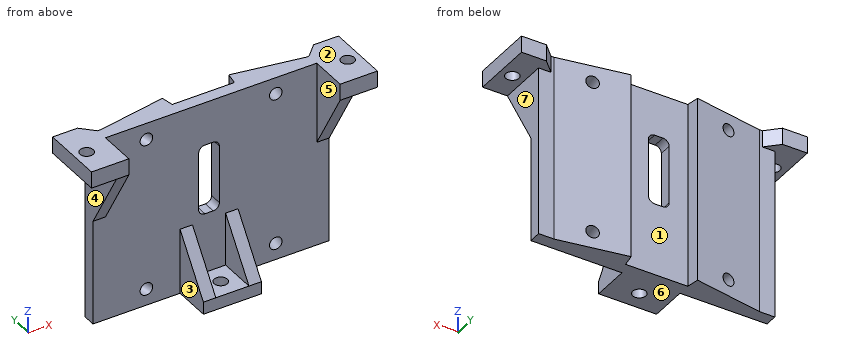
from build123d import *

# Parameters (mm, degrees)
SKETCH_1_W          = 57
SKETCH_1_H          = 45
EXTRUDE_1_DEPTH     = 3
SKETCH_2_W          = 4
SKETCH_2_H          = 15
EXTRUDE_2_DEPTH     = 6
SKETCH_3_W          = 4
SKETCH_3_H          = 15
EXTRUDE_3_DEPTH     = 6
EXTRUDE_4_DEPTH     = 3
SKETCH_5_W          = 4
SKETCH_5_H          = 9
EXTRUDE_5_DEPTH     = 3
CHAMFER_1_SIZE      = 3
SKETCH_6_R          = 1.6
CUT_EXTRUDE_1_DEPTH = 4
SKETCH_8_W          = 8
SKETCH_8_H          = 3
EXTRUDE_6_DEPTH     = 9
EXTRUDE_7_DEPTH     = 3
EXTRUDE_8_DEPTH     = 3
SKETCH_11_R         = 1.6
CUT_EXTRUDE_3_DEPTH = 3
SKETCH_12_W         = 5
SKETCH_12_H         = 17
CUT_EXTRUDE_4_DEPTH = 3
FILLET_1_R          = 1.5
EXTRUDE_9_REACH     = 80.57
SKETCH_15_W         = 45
SKETCH_15_H         = 17.726539555
SKETCH_16_R         = 1.5
CUT_EXTRUDE_5_DEPTH = 79.570276896


with BuildPart() as part:
    # 草图1 → 凸台-拉伸1 (new body)
    with BuildSketch(Plane(origin=(0, 0, 0), x_dir=(1, 0, 0), z_dir=(0, 1, 0))):
        with Locations((28.5, 22.5)):
            Rectangle(SKETCH_1_W, SKETCH_1_H)
    extrude(amount=EXTRUDE_1_DEPTH)

    # 草图2 → 凸台-拉伸2 (add)
    with BuildSketch(Plane.ZY):
        with Locations((-2, -1.5)):
            Rectangle(SKETCH_2_W, SKETCH_2_H)
    extrude(amount=EXTRUDE_2_DEPTH)

    # 草图3 → 凸台-拉伸3 (add)
    with BuildSketch(Plane(origin=(57, 0, 0), x_dir=(0, 0, -1), z_dir=(1, 0, 0))):
        with Locations((2, -1.5)):
            Rectangle(SKETCH_3_W, SKETCH_3_H)
    extrude(amount=EXTRUDE_3_DEPTH)

    # 草图4 → 凸台-拉伸4 (add)
    with BuildSketch(Plane.ZY.offset(-57)):
        Polygon((-4, -9), (-19.588457268, 0), (0, 0), (0, -9), align=None)
    extrude(amount=EXTRUDE_4_DEPTH)

    # 草图5 → 凸台-拉伸5 (add)
    with BuildSketch(Plane(origin=(0, 0, 0), x_dir=(0, 0, -1), z_dir=(1, 0, 0))):
        Polygon((19.588457268, 0), (4, 0), (4, -9), align=None)
        with Locations((2, -4.5)):
            Rectangle(SKETCH_5_W, SKETCH_5_H)
    extrude(amount=EXTRUDE_5_DEPTH)

    # 倒角1
    chamfer_1_edges = [part.edges().sort_by_distance(p)[0] for p in [
        (0, 3, -2),
        (57, 3, -2),
    ]]
    chamfer(chamfer_1_edges, length=CHAMFER_1_SIZE - 0.0001)  # a hair under: the kernel refuses the full size

    # 草图6 → 切除-拉伸1 (cut)
    with BuildSketch(Plane(origin=(0, 0, -4), x_dir=(-1, 0, 0), z_dir=(0, 0, -1))):
        with Locations(Location((3, -2.323268139, 0), (0, 0, 90))):
            Circle(SKETCH_6_R)
        with Locations(Location((-60, -2.323268139, 0), (0, 0, 90))):
            Circle(SKETCH_6_R)
    extrude(amount=-CUT_EXTRUDE_1_DEPTH, mode=Mode.SUBTRACT)

    # 草图8 → 凸台-拉伸6 (add)
    with BuildSketch(Plane.XZ):
        with Locations((28, -43.5)):
            Rectangle(SKETCH_8_W, SKETCH_8_H)
    extrude(amount=EXTRUDE_6_DEPTH)

    # 草图9 → 凸台-拉伸7 (add)
    with BuildSketch(Plane(origin=(32, 0, 0), x_dir=(0, 0, -1), z_dir=(1, 0, 0))):
        Polygon((45, 0), (29.146667939, 0), (42, -9), (45, -9), align=None)
    extrude(amount=EXTRUDE_7_DEPTH)

    # 草图10 → 凸台-拉伸8 (add)
    with BuildSketch(Plane.ZY.offset(-24)):
        Polygon((-45, 0), (-45, -9), (-42, -9), (-29.146667939, 0), align=None)
    extrude(amount=EXTRUDE_8_DEPTH)

    # 草图11 → 切除-拉伸3 (cut)
    with BuildSketch(Plane.XY.offset(-42)):
        with Locations((28, -4.5)):
            Circle(SKETCH_11_R)
    extrude(amount=-CUT_EXTRUDE_3_DEPTH, mode=Mode.SUBTRACT)

    # 草图12 → 切除-拉伸4 (cut)
    with BuildSketch(Plane(origin=(0, 3, 0), x_dir=(1, 0, 0), z_dir=(0, 1, 0))):
        with Locations((28, 19)):
            Rectangle(SKETCH_12_W, SKETCH_12_H)
    extrude(amount=-CUT_EXTRUDE_4_DEPTH, mode=Mode.SUBTRACT)

    # 圆角1
    fillet_1_edges = [part.edges().sort_by_distance(p)[0] for p in [
        (25.5, 1.5, -27.5),
        (30.5, 1.5, -27.5),
        (30.5, 1.5, -10.5),
        (25.5, 1.5, -10.5),
    ]]
    fillet(fillet_1_edges, radius=FILLET_1_R)

    # 草图15 → 凸台-拉伸9 (add, up to next)
    with BuildSketch(Plane(origin=(2.119507574, 12.02032477, 0), x_dir=(0, 0, 1), z_dir=(0.17364817766693066, 0.9848077530122081, 0)), mode=Mode.PRIVATE) as extrude_9_sk1:
        with Locations((-22.5, 43.795404353)):
            Rectangle(SKETCH_15_W, SKETCH_15_H)
    extrude_9_tool1 = extrude(extrude_9_sk1.sketch, amount=-EXTRUDE_9_REACH, mode=Mode.PRIVATE) - part.part
    extrude_9 = extrude_9_tool1.solids().sort_by_distance((45.249561, 4.415333, -22.5))[0]
    add(extrude_9)

    # 草图16 → 切除-拉伸5 (cut, through all)
    with BuildSketch(Plane(origin=(2.119507574, 12.02032477, 0), x_dir=(0.9848077530122081, -0.17364817766693064, 0), z_dir=(0.17364817766693064, 0.9848077530122081, 0))):
        with Locations(Location((43.439057305, 41, 0), (0, 0, 180))):
            Circle(SKETCH_16_R)
        with Locations((43.439057305, 4)):
            Circle(SKETCH_16_R)
    cut_extrude_5 = extrude(amount=-CUT_EXTRUDE_5_DEPTH, mode=Mode.SUBTRACT)

    # 镜向1: 凸台-拉伸9, 切除-拉伸5 across plane
    add(extrude_9.mirror(Plane(origin=(28.5, 0, 0), x_dir=(0, 0, 1), z_dir=(1, 0, 0))))
    add(cut_extrude_5.mirror(Plane(origin=(28.5, 0, 0), x_dir=(0, 0, 1), z_dir=(1, 0, 0))), mode=Mode.SUBTRACT)


solid = part.part
Geometry check sheet. Reference: the model listing, model coordinates, mm. Face numbers are marked on the shaded views. A direction names the side the tool comes from. Give positions to 0.01 mm unless a question says otherwise; leave off trailing zeros. Loops run counter-clockwise (first coordinate to the right, second up) from the corner with the lowest first, then second, coordinate; pieces in that order, holes last. Notation, with made-up numbers: M 21,37.25 L 50,37.25 A24 ccw 50,57.25 Z; hole C 88.5,-23 d10. An arc over 180 degrees is marked long. Answer as a JSON object with one key per item and string values. Group by question number.
Item 1: Sectioned sample at A-A on x = 28. Record the boundary of the cut face in (y, z).
Item 2: Access from +Z, -Z, +X, -X, +Y, -Y to the whole of each face (thin tool, end or side, straight path). Record for the marked faces 1, 2, 3 and 4.
Item 3: Sectioned sample at C-C on z = -35.5. Record the boundary of the cut face in (x, y).
Item 4: Sectioned sample at D-D on z = -30. Record the boundary of the cut face in (x, y).
Item 5: Material ranges on L1, parallel to X at y = 0.5, z = -20.5; L2, parallel to X at y = -1.75, z = -14; L3, parallel to Z at x = 14, y = 0.75, recorded low to high.
Item 6: Gauge pin test, flat ends, axial feed: pin 1 (4.5 mm diameter, centred on y = -5, z = -7, fed in from +X); pin 2 (1.5 mm diameter, centred on x = 7, z = -32.5, fed in from +Y); pin 3 (10 mm diameter, centred on x = 44.5, z = -38.5, fed in from +Y); pin 4 (3 mm diameter, centred on x = 14, y = -3, fed in from -Z). Record the tip position at first contact, or that the pin passes through.
Item 7: Sectioned sample at B-B on x = -3. Record the boundary of the cut face in (y, z), plus the area to 3 significant figures.
Item 8: Mould release check, pull along X, two halves, no side actions. Record for the marked faces 5, 6 and 7: pulls with the +X half, pulls with the -X half, needs draft (parallel to the pull), parting line crosses it, or undercut.
Findings below:
{
 "1": {"outline": "M -9,-45 L -6.1,-45 L -6.1,-42 L -9,-42 Z; M -2.9,-45 L 3,-45 L 3,-27.5 L 0,-27.5 L 0,-42 L -2.9,-42 Z; M 0,-10.5 L 3,-10.5 L 3,0 L 0,0 Z"},
 "2": {"face 1": "+Z, -Z, +Y", "face 2": "+Z, +X, -X, +Y, -Y", "face 3": "+Z, -Z, -X, -Y", "face 4": "-Z, -X, +Y, -Y"},
 "3": {"outline": "M 0,0 L 21,0 L 21,-4.45 L 24,-4.45 L 24,0 L 32,0 L 32,-4.45 L 35,-4.45 L 35,0 L 57,0 L 57,3 L 53.28,3 L 36.52,5.95 L 36,3 L 21,3 L 20.48,5.95 L 3.72,3 L 0,3 Z"},
 "4": {"outline": "M 0,0 L 21,0 L 21,-0.6 L 24,-0.6 L 24,0 L 32,0 L 32,-0.6 L 35,-0.6 L 35,0 L 57,0 L 57,3 L 53.28,3 L 36.52,5.95 L 36,3 L 21,3 L 20.48,5.95 L 3.72,3 L 0,3 Z"},
 "5": {"L1": "0 to 25.5, 30.5 to 57", "L2": "0 to 3, 54 to 57", "L3": "-45 to -41.87, -40.13 to -4.87, -3.13 to 0"},
 "6": {"pin 1": "x = 57", "pin 2": "y = 3.71", "pin 3": "y = 5.43", "pin 4": "through"},
 "7": {"outline": "M -9,-4 L -3.92,-4 L -3.92,0 L -9,0 Z; M -0.72,-4 L 6,-4 L 6,0 L -0.72,0 Z", "area": "47.2 mm2"},
 "8": {"face 5": "undercut", "face 6": "needs draft", "face 7": "pulls with the +X half"}
}
